Answer from the drawing. Dimensions are ordinates in mm from the lowest x, y and z of the part. Give positions to 0.01 mm unless a question says otherwise; leave off trailing zeros. Loops run counter-clockwise (first coordinate to the right, second up) from the corner with the lowest first, then second, coordinate; pieces in that order, holes last. Notation, with made-up numbers: M 9,69 L 50,69 A29 ccw 50,102 Z; hole C 65.25,-27.5 d4. An arc over 180 degrees is marked long. Use a Markdown table: item, result.
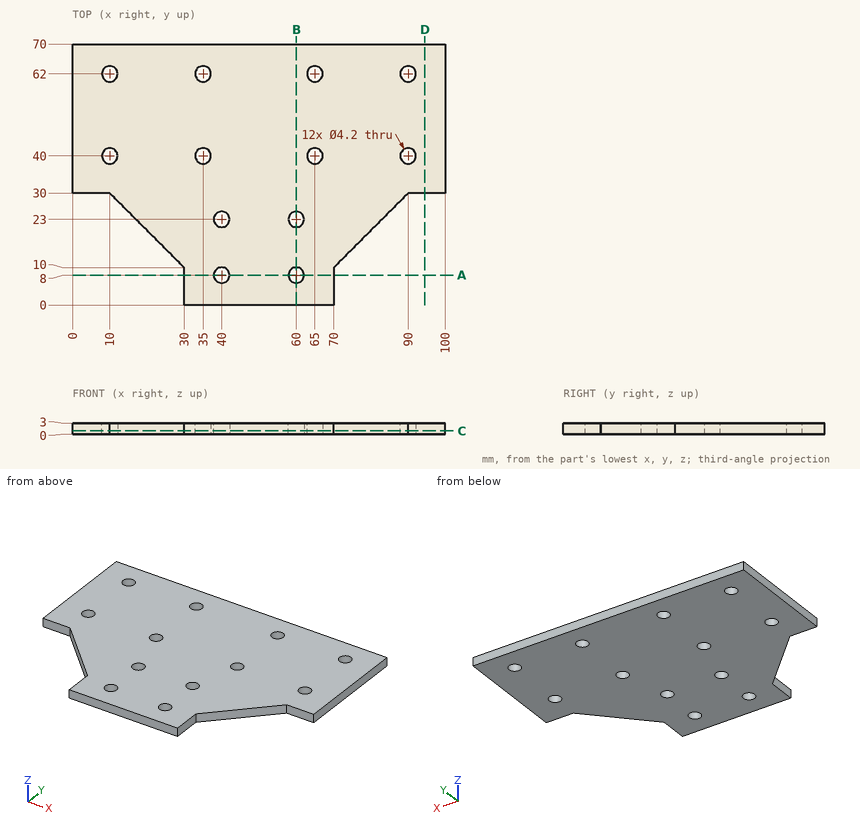
(1) A cutting plane is placed at D-D (x = 94.5). Write down the section's boundary in (y, z).
Entries:
| item | result |
|---|---|
| outline | M 30,0 L 70,0 L 70,3 L 30,3 Z |
(2) A cutting plane is placed at B-B (x = 60). Write down the section's boundary in (y, z).
Entries:
| item | result |
|---|---|
| outline | M 0,0 L 5.9,0 L 5.9,3 L 0,3 Z; M 10.1,0 L 20.9,0 L 20.9,3 L 10.1,3 Z; M 25.1,0 L 70,0 L 70,3 L 25.1,3 Z |
(3) Given P1, Ø5.5, axis at x = 10, y = 62, coming from the +Z side; P2, Ø0.9, axis at y = 6, z = 1.5, coming from the -X side; P3, Ø0.9, axis at x = 95.5, z = 2, coming from the -Y side, each flat-ended and moving along its own axis, determine where each tip first touches the part or whether it passes through.
Entries:
| item | result |
|---|---|
| P1 | stops at z = 3 |
| P2 | stops at x = 30 |
| P3 | stops at y = 30 |
(4) A cutting plane is placed at A-A (y = 8). Write down the section's boundary in (x, z), and give its area (3 significant figures).
Entries:
| item | result |
|---|---|
| outline | M 30,0 L 37.9,0 L 37.9,3 L 30,3 Z; M 42.1,0 L 57.9,0 L 57.9,3 L 42.1,3 Z; M 62.1,0 L 70,0 L 70,3 L 62.1,3 Z |
| area | 94.8 mm² |
(5) Consider probe 1 along Y at (x, z) = (65, 0.8); probe 2 along Y at (x, z) = (60, 0.7); probe 3 along X at (y, z) = (5, 2.45). Determine where each line is inside the solid, lowest interval first. Write a range as [from, to].
Entries:
| item | result |
|---|---|
| probe 1 | y = [0, 37.9], [42.1, 59.9], [64.1, 70] |
| probe 2 | y = [0, 5.9], [10.1, 20.9], [25.1, 70] |
| probe 3 | x = [30, 70] |
(6) A cutting plane is placed at C-C (z = 0.9). Count the separate pieces of the cut face and the enclosed holes in it, and give its area (3 significant figures).
Entries:
| item | result |
|---|---|
| separate pieces | 1 |
| enclosed holes | 12 |
| area | 5,430 mm² |
